```python
from build123d import *

# Parameters (mm, degrees)
F0_R     = 1.905
F1_DEPTH = 4.318
F2_SIZE  = 0.508


with BuildPart() as f1:
    # F0 (on Top) → F1 (new body)
    with BuildSketch(Plane.XY):
        Polygon((-31.75, -88.9), (31.75, -88.9), (31.75, 88.9), (-31.75, 88.9), (-31.75, -30.1498), (-12.7, -30.1498), (-12.7, -46.0248), (-31.75, -46.0248), align=None)
        with Locations((-15.875, -63.5)):
            Circle(F0_R, mode=Mode.SUBTRACT)
        with Locations((15.875, -63.5)):
            Circle(F0_R, mode=Mode.SUBTRACT)
        with Locations((-15.875, 0)):
            Circle(F0_R, mode=Mode.SUBTRACT)
        with Locations((-15.875, 63.5)):
            Circle(F0_R, mode=Mode.SUBTRACT)
        with Locations((15.875, 0)):
            Circle(F0_R, mode=Mode.SUBTRACT)
        with Locations((15.875, 63.5)):
            Circle(F0_R, mode=Mode.SUBTRACT)
    extrude(amount=F1_DEPTH)

    # F2
    f2_edges = [f1.edges().sort_by_distance(p)[0] for p in [
        (0, -88.9, 0),
        (-31.75, -67.4624, 0),
        (-22.225, -46.0248, 0),
        (-12.7, -38.0873, 0),
        (-22.225, -30.1498, 0),
        (-31.75, 29.3751, 0),
        (0, 88.9, 0),
        (31.75, 0, 0),
        (-17.78, 0, 0),
        (13.97, 0, 0),
        (13.97, -63.5, 0),
        (-17.78, -63.5, 0),
        (-17.78, 63.5, 0),
        (13.97, 63.5, 0),
    ]]
    chamfer(f2_edges, length=F2_SIZE)


solid = f1.part
```
Geometry: final body of the model. Coordinates: model frame, mm. A direction names the side the tool comes from. Coordinates: 2 decimals unless noted, no trailing zeros. Order: outer loops, then holes, each group sorted by start corner. A loop starts at its lowest first (then second) coordinate and runs counter-clockwise, first axis right, second up. Notation, with made-up numbers: M -13.5,87.5 L 1.5,87.5 A11 ccw 1.5,95.5 Z; hole C -10,-7 d10. An arc over 180 degrees is marked long. Answer in a Markdown table with one row per item. Add a question column.
Q1. Contact query for a flat-ended pin moving along its axis: P1, Ø3.5, axis at x = 15.875, y = 0, coming from the +Z side. Output: stop coordinate, or through.
Q2. Section query B-B on x = -23.5. Return the cut outline in (y, z), and give its area (3 significant figures).
Q3. Mould query, pull axis X, two halves, no side actions, for faces 3 (the flat face through (-22, -46.025, 2)), 4 (the cylindrical face through (17.635, -0.73, 2.386)), 5 (the flat face through (-31.75, -67, 2)). Classes: released by +X, released by -X, zero draft, split by the parting line, or undercut.
Q4. Reachability of faces 1 (the flat face through (-12.7, -38, 2)), 2 (the cylindrical face through (-14.115, -0.73, 2.386)) from +Z, -Z, +X, -X, +Y, -Y: full face, straight path, thin tool, end or side. Return the list, or none.
Q5. Section query A-A on y = 0. Return the cut outline in (x, z), and give its area (3 significant figures).
Q6. Section query D-D on y = -44.5. Return the cut outline in (x, z), and give its area (3 significant figures).
Q7. Line query: L1, parallel to Y at x = -19.5, z = 1.35; L2, parallel to Y at x = 17, z = 1.25; L3, parallel to Y at x = 17.5, z = 1.4. Output: solid intervals per line, ascending.
Q8. Section query C-C on z = 1.65. Return the cut outline in (x, y) (3 decimals).
Completed:
| question | item | result |
|---|---|---|
| 1 | P1 | passes through |
| 2 | outline | M -88.9,0.51 L -88.39,0 L -46.53,0 L -46.02,0.51 L -46.02,4.32 L -88.9,4.32 Z; M -30.15,0.51 L -29.64,0 L 88.39,0 L 88.9,0.51 L 88.9,4.32 L -30.15,4.32 Z |
| 2 | area | 699 mm2 |
| 3 | face 3 | zero draft |
| 3 | face 4 | undercut |
| 3 | face 5 | released by -X |
| 4 | face 1 | +Z, -Z, -X |
| 4 | face 2 | +Z, -Z |
| 5 | outline | M -31.75,0.51 L -31.24,0 L -18.29,0 L -17.78,0.51 L -17.78,4.32 L -31.75,4.32 Z; M -13.97,0.51 L -13.46,0 L 13.46,0 L 13.97,0.51 L 13.97,4.32 L -13.97,4.32 Z; M 17.78,0.51 L 18.29,0 L 31.24,0 L 31.75,0.51 L 31.75,4.32 L 17.78,4.32 Z |
| 5 | area | 241 mm2 |
| 6 | outline | M -12.7,0.51 L -12.19,0 L 31.24,0 L 31.75,0.51 L 31.75,4.32 L -12.7,4.32 Z |
| 6 | area | 192 mm2 |
| 7 | L1 | y = -88.9 to -46.02, -30.15 to 88.9 |
| 7 | L2 | y = -88.9 to -65.04, -61.96 to -1.54, 1.54 to 61.96, 65.04 to 88.9 |
| 7 | L3 | y = -88.9 to -64.49, -62.51 to -0.99, 0.99 to 62.51, 64.49 to 88.9 |
| 8 | outline | M -31.75,-88.9 L 31.75,-88.9 L 31.75,88.9 L -31.75,88.9 L -31.75,-30.15 L -12.7,-30.15 L -12.7,-46.025 L -31.75,-46.025 Z; hole C -15.875,-63.5 d3.81; hole C -15.875,0 d3.81; hole C -15.875,63.5 d3.81; hole C 15.875,-63.5 d3.81; hole C 15.875,0 d3.81; hole C 15.875,63.5 d3.81 |
